```python
from build123d import *

# Parameters (mm, degrees)
F0_W     = 390
F0_H     = 800
F1_DEPTH = 10
F3_DEPTH = 25
F5_D     = 8.8


with BuildPart() as f1:
    # F0 (on Front) → F1 (new body)
    with BuildSketch(Plane.XZ):
        Rectangle(F0_W, F0_H)
    extrude(amount=F1_DEPTH)

    # F2 (on face) → F3 (cut)
    with BuildSketch(Plane.XZ.offset(10)):
        Polygon((5, -190), (195, -320), (195, 400), (-95, 400), (5, 300), align=None)
    extrude(amount=-F3_DEPTH, mode=Mode.SUBTRACT)

    # F5 (through all)
    with Locations(Plane.XZ.offset(10)):
        with Locations((-130, 160), (-60, 160), (-130, -80), (-60, -80), (-130, -340), (0, -340), (130, -340)):
            Hole(F5_D / 2)


solid = f1.part
```
Geometry check sheet. Reference: the model listing, model coordinates, mm. Give positions to 0.01 mm unless a question says otherwise; leave off trailing zeros. Order: outer loops, then holes, each group sorted by start corner. A loop starts at its lowest first (then second) coordinate and runs counter-clockwise, first axis right, second up. Notation, with made-up numbers: (-35.5, 31.25) - (17.5, 31.25) arc R18 ccw to (17.5, 56.25) - close; hole circle Ø8 at (-13.5, 1). An arc over 180 degrees is marked (long way). Answer in a Markdown table with one row per item. Add a question column.
Q1. Cross-section at B-B, the plane z = 283.5. Enter the section's corners in (x, y).
Q2. Material ranges on probe 1 along Z at (x, y) = (-130, -6); probe 2 along X at (y, z) = (-5, -340); probe 3 along X at (y, z) = (-2.25, 159), recorded low to high. Write a range as from..to.
Q3. Cross-section at C-C, the plane x = 157. Enter the section's corners in (y, z), then the cut area to 3 significant figures.
Q4. Cross-section at A-A, the plane y = -2. Enter the section's corners in (x, z), then the cut area to 3 significant figures.
Q5. Gauge pin test, flat ends, axial feed: pin 1 (8 mm diameter, centred on x = -130, z = -340, fed in from -Y); pin 2 (5 mm diameter, centred on y = -3.5, z = 125.5, fed in from +X); pin 3 (1.5 mm diameter, centred on x = 113, y = -5.5, fed in from +Z); pin 4 (11.5 mm diameter, centred on x = 130, z = -340, fed in from +Y). Record the tip position at first contact, or that the pin passes through.
Check values:
| question | item | result |
|---|---|---|
| 1 | outline | (-195, -10) - (5, -10) - (5, 0) - (-195, 0) - close |
| 2 | probe 1 | z = -400..-344.4, -335.6..-84.4, -75.6..155.6, 164.4..400 |
| 2 | probe 2 | x = -195..-134.4, -125.6..-4.4, 4.4..125.6, 134.4..195 |
| 2 | probe 3 | x = -195..-134.28, -125.72..-64.28, -55.72..5 |
| 3 | outline | (-10, -400) - (0, -400) - (0, -294) - (-10, -294) - close |
| 3 | area | 1,060 mm^2 |
| 4 | outline | (-195, -400) - (195, -400) - (195, -320) - (5, -190) - (5, 300) - (-95, 400) - (-195, 400) - close; hole circle Ø8.8 at (-130, -340); hole circle Ø8.8 at (-130, -80); hole circle Ø8.8 at (-130, 160); hole circle Ø8.8 at (-60, -80); hole circle Ø8.8 at (-60, 160); hole circle Ø8.8 at (0, -340); hole circle Ø8.8 at (130, -340) |
| 4 | area | 182,000 mm^2 |
| 5 | pin 1 | passes through |
| 5 | pin 2 | stops at x = 5 |
| 5 | pin 3 | stops at z = -263.38 |
| 5 | pin 4 | stops at y = 0 |
